Geometry: final body of the model. Coordinates: model frame, mm. A direction names the side the tool comes from. Round coordinates to 2 decimals unless told otherwise and drop trailing zeros. Loops run counter-clockwise (first coordinate to the right, second up) from the corner with the lowest first, then second, coordinate; pieces in that order, holes last. Notation, with made-up numbers: (-8, 89) - (37, 89) arc R24 cw to (37, 118) - close; hole circle Ø7 at (42, 55). An arc over 180 degrees is marked (long way). Answer in a Markdown table with one row per item. Add a question column.
from build123d import *

# Parameters (mm, degrees)
F1_DEPTH = 90
F2_R     = 3
F3_R     = 6


with BuildPart() as f1:
    # F0 (on Top) → F1 (new body)
    with BuildSketch(Plane.XY):
        Polygon((93, 38.521861), (38.521861, 93), (-38.521861, 93), (-93, 38.521861), (-93, -38.521861), (-38.521861, -93), (38.521861, -93), (93, -38.521861), align=None)
        Polygon((-90, 37.279221), (-37.279221, 90), (37.279221, 90), (90, 37.279221), (90, -37.279221), (37.279221, -90), (-37.279221, -90), (-90, -37.279221), align=None, mode=Mode.SUBTRACT)
    extrude(amount=F1_DEPTH)

    # F2
    f2_edges = [f1.edges().sort_by_distance(p)[0] for p in [
        (-37.279221, 90, 45),
        (37.279221, 90, 45),
        (90, 37.279221, 45),
        (90, -37.279221, 45),
        (37.279221, -90, 45),
        (-37.279221, -90, 45),
        (-90, -37.279221, 45),
        (-90, 37.279221, 45),
    ]]
    fillet(f2_edges, radius=F2_R)

    # F3
    f3_edges = [f1.edges().sort_by_distance(p)[0] for p in [
        (-93, -38.521861, 45),
        (-38.521861, -93, 45),
        (38.521861, -93, 45),
        (93, -38.521861, 45),
        (93, 38.521861, 45),
        (38.521861, 93, 45),
        (-38.521861, 93, 45),
        (-93, 38.521861, 45),
    ]]
    fillet(f3_edges, radius=F3_R)


solid = f1.part
1) Reachability of faces 1 (the flat face through (90, 1, 44)), 2 (the cylindrical face through (38.36, -92.53, 45.63)) from +Z, -Z, +X, -X, +Y, -Y: full face, straight path, thin tool, end or side. Return the list, or none.
2) Contact query for flat-ended pins moving along their axis: pin 1 Ø5 at (x, z) = (-45, 21) entering from -Y; pin 2 Ø3 at (y, z) = (-43, 38) entering from -X; pin 3 Ø6 at (x, y) = (73, 51) entering from -Z; pin 4 Ø1.5 at (y, z) = (50.5, 71.5) entering from +X. Output: stop coordinate, or through.
3) Section A-A, the plane x = 12. Return the cut outline in (y, z), and give its area (3 significant figures).
4) Pull-direction query (Y, two-part tool) for faces 3 (the cylindrical face through (-92.556, -38.302, 45.63)), 4 (the flat face through (1, 93, 44)), 5 (the flat face through (63.28, 64, 44.37)); classes: pulls with the +Y half, pulls with the -Y half, needs draft (parallel to the pull), parting line crosses it, or undercut.
5) Material intervals for line 1 along X through (y, z) = (-14, 38.5); line 2 along X through (y, z) = (37, 28), sorted ascending. Write a range as from..to.
Evaluation:
| question | item | result |
|---|---|---|
| 1 | face 1 | +Z, -Z |
| 1 | face 2 | +Z, -Z, +X, -Y |
| 2 | pin 1 | stops at y = -89.02 |
| 2 | pin 2 | stops at x = -90.02 |
| 2 | pin 3 | stops at z = 0 |
| 2 | pin 4 | stops at x = 81.77 |
| 3 | outline | (-93, 0) - (-90, 0) - (-90, 90) - (-93, 90) - close; (90, 0) - (93, 0) - (93, 90) - (90, 90) - close |
| 3 | area | 540 mm² |
| 4 | face 3 | pulls with the -Y half |
| 4 | face 4 | pulls with the +Y half |
| 4 | face 5 | undercut |
| 5 | line 1 | x = -93..-90, 90..93 |
| 5 | line 2 | x = -92.92..-89.84, 89.84..92.92 |
